For this review, use the dimensioned drawing (mm, ordinates from the lowest corner) and the shaded views. Give positions to 0.01 mm unless a question says otherwise; leave off trailing zeros. Write each loop counter-clockwise with the first axis right and the second up, starting at its lowest first coordinate (ties: lowest second). Pieces come first, ordered by that corner, then holes. Notation, with made-up numbers: (45, -17.75) - (85, -17.75) arc R15 ccw to (85, 6.25) - close; hole circle Ø2 at (31.25, -30.75). An arc over 180 degrees is marked (long way). Use a Markdown table: item, result. Add a question column.
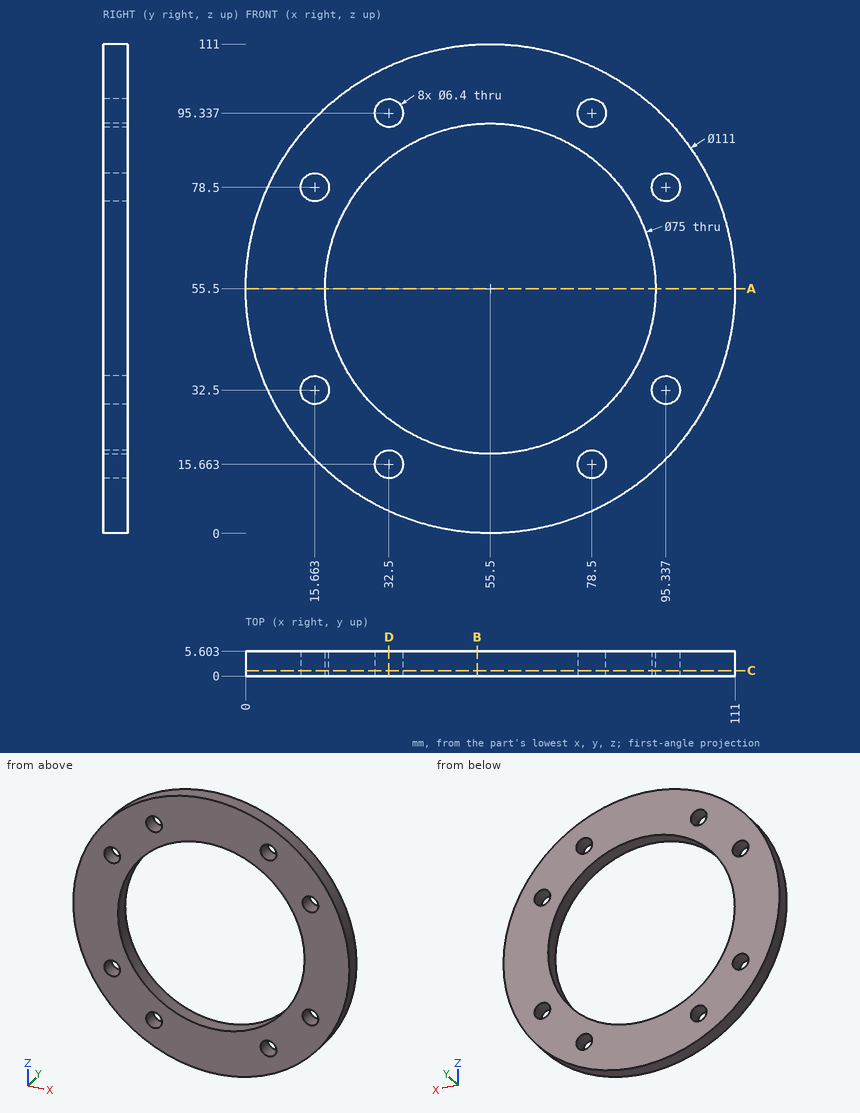
(1) Add section A-A (z = 55.5). State the section outline as (x, y) points.
(2) Insertion check: pin 1 (1.5 mm diameter, centred on y = 2.5, z = 29.5, fed in from -X); pin 2 (2 mm diameter, centred on y = 1, z = 64.5, fed in from -X); pin 3 (1.5 mm diameter, centred on x = 73, y = 3, fed in from +Z). Each pin has a flat end and moves straight along its axis. Give the tip position at first contact, or say it passes through.
(3) Add section C-C (y = 1.2). Count the separate pieces of the cut face and the enclosed holes in it, and give its area (3 significant figures).
(4) Add section B-B (x = 52.5). State the section outline as (y, z) points.
(5) For line 1 along X through (y, z) = (1.85, 55.5); line 2 along X through (y, z) = (0.4, 34) (1 decimal); line 3 along Z through (x, y) = (32.5, 4.3), list the stretches that pass through material, from the lowest coordinate up.
(6) Add section D-D (x = 32.5). State the section outline as (y, z) points.
Answers follow:
| question | item | result |
|---|---|---|
| 1 | outline | (0, 0) - (18, 0) - (18, 5.6) - (0, 5.6) - close; (93, 0) - (111, 0) - (111, 5.6) - (93, 5.6) - close |
| 2 | pin 1 | x = 6.08 |
| 2 | pin 2 | x = 0.58 |
| 2 | pin 3 | z = 108.41 |
| 3 | separate pieces | 1 |
| 3 | enclosed holes | 9 |
| 3 | area | 5,000 mm^2 |
| 4 | outline | (0, 0.08) - (5.6, 0.08) - (5.6, 18.12) - (0, 18.12) - close; (0, 92.88) - (5.6, 92.88) - (5.6, 110.92) - (0, 110.92) - close |
| 5 | line 1 | 0 to 18, 93 to 111 |
| 5 | line 2 | 4.3 to 12.8, 18.5 to 24.8, 86.2 to 92.5, 98.2 to 106.7 |
| 5 | line 3 | 4.99 to 12.46, 18.86 to 25.88, 85.12 to 92.14, 98.54 to 106.01 |
| 6 | outline | (0, 4.99) - (5.6, 4.99) - (5.6, 12.46) - (0, 12.46) - close; (0, 18.86) - (5.6, 18.86) - (5.6, 25.88) - (0, 25.88) - close; (0, 85.12) - (5.6, 85.12) - (5.6, 92.14) - (0, 92.14) - close; (0, 98.54) - (5.6, 98.54) - (5.6, 106.01) - (0, 106.01) - close |
